Can you work these out from the model? Positions are in its coordinate system, mm. Face numbers are marked on the shaded views. Coordinates: 2 decimals unless noted, no trailing zeros. Loops run counter-clockwise (first coordinate to the right, second up) from the corner with the lowest first, then second, coordinate; pieces in that order, holes last.
```python
from build123d import *

# Parameters (mm, degrees)
SKETCH_1_W          = 800
SKETCH_1_H          = 20
SKETCH_1_R          = 6
EXTRUDE_1_DEPTH     = 500
SKETCH_5_R          = 15
CUT_EXTRUDE_2_DEPTH = 814.854186619
SKETCH_6_W          = 40
SKETCH_6_H          = 400
CUT_EXTRUDE_3_DEPTH = 816.389199244


with BuildPart() as part:
    # 草图1 → 凸台-拉伸1 (new body)
    # profile 1 of 3: a face of its own
    with BuildSketch(Plane.XY):
        Rectangle(SKETCH_1_W, SKETCH_1_H)
    # profile 2 of 3: a face of its own
    with BuildSketch(Plane.XY):
        with BuildLine():
            ThreePointArc((-600, -10), (-500, -42.522729151), (-400, -10))
            Line((-400, -10), (-400, 10))
            ThreePointArc((-400, 10), (-500, -22.522729151), (-600, 10))
            Line((-600, 10), (-600, -10))
        make_face()
    # profile 3 of 3: a face of its own
    with BuildSketch(Plane.XY):
        Polygon((-640, -10), (-600, -10), (-600, 10), (-600, 30), (-640, 30), align=None)
        with Locations((-620, 10)):
            Circle(SKETCH_1_R, mode=Mode.SUBTRACT)
    extrude(amount=EXTRUDE_1_DEPTH)

    # 草图5 → 切除-拉伸2 (cut, through all)
    with BuildSketch(Plane(origin=(0, 10, 0), x_dir=(1, 0, 0), z_dir=(0, 1, 0))):
        with Locations(Location((-300, -440, 0), (0, 0, 180))):
            Circle(SKETCH_5_R)
        with Locations(Location((-300, -60, 0), (0, 0, 180))):
            Circle(SKETCH_5_R)
    extrude(amount=-CUT_EXTRUDE_2_DEPTH, mode=Mode.SUBTRACT)

    # 草图6 → 切除-拉伸3 (cut, through all)
    with BuildSketch(Plane(origin=(0, 30, 0), x_dir=(1, 0, 0), z_dir=(0, 1, 0))):
        with Locations((-620, -250)):
            Rectangle(SKETCH_6_W, SKETCH_6_H)
    extrude(amount=-CUT_EXTRUDE_3_DEPTH, mode=Mode.SUBTRACT)


solid = part.part
```
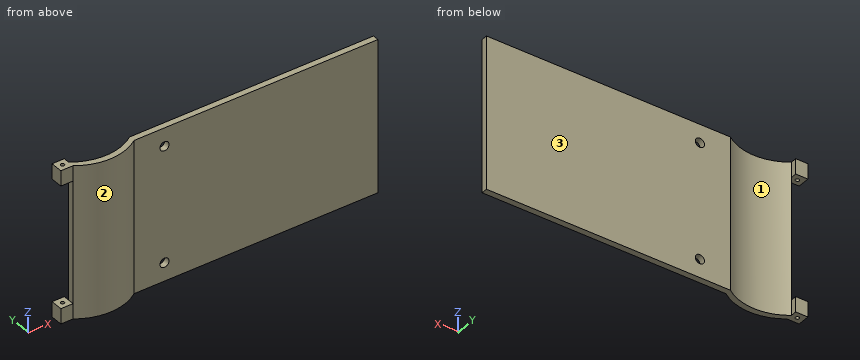
Item 1: I need wall thicknesses on line 1 along Z through (x, y) = (-300, -4); line 2 along Y through (x, z) = (-620, 466.5); line 3 along X through (y, z) = (9.5, 156.5). Which ranges of each line are inside material? Lowest first, please.
Results are:
line 1: z = 0 to 45, 75 to 425, 455 to 500
line 2: y = -10 to 4, 16 to 30
line 3: x = -600 to -599.31, -400.69 to 400
Item 2: Suppose I cut it at A-A, the plane z = 60. Please give me the cut outline in (x, y), plus the area to 3 significant figures.
Results are:
outline: (-600, -10) arc R170 ccw to (-400, -10) - (-315, -10) - (-315, 10) - (-400, 10) arc R170 cw to (-600, 10) - close; (-285, -10) - (400, -10) - (400, 10) - (-285, 10) - close
area: 19,400 mm2
Item 3: We'd pull the mould along X, two halves only. Please class the marked faces 1, 2 and 3: +X half, -X half, draft (parallel to the pull), parting line (faces both ways), or undercut.
Results are:
face 1: undercut
face 2: parting line
face 3: draft
Item 4: Suppose I cut it at C-C, the plane z = 286. Please give me the cut outline in (x, y), plus the area to 3 significant figures.
Results are:
outline: (-600, -10) arc R170 ccw to (-400, -10) - (400, -10) - (400, 10) - (-400, 10) arc R170 cw to (-600, 10) - close
area: 20,000 mm2
Item 5: Suppose I cut it at B-B, the plane x = -300. Please give me the cut outline in (y, z).
Results are:
outline: (-10, 0) - (10, 0) - (10, 45) - (-10, 45) - close; (-10, 75) - (10, 75) - (10, 425) - (-10, 425) - close; (-10, 455) - (10, 455) - (10, 500) - (-10, 500) - close
Item 6: I'm going to push flat-ended pins straight in: P1, Ø22, axis at y = -4.5, z = 284, coming from the -X side; P2, Ø10, axis at y = 21, z = 465.5, coming from the +X side; P3, Ø3, axis at x = -67.5, z = 356, coming from the +Y side. Where does each tip first touch, or does it pass through?
Results are:
P1: stops at x = -600
P2: stops at x = -600
P3: stops at y = 10
Item 7: Suppose I cut it at D-D, the plane x = 93. Please give me the cut outline in (y, z), plus the area to 3 significant figures.
Results are:
outline: (-10, 0) - (10, 0) - (10, 500) - (-10, 500) - close
area: 10,000 mm2
